from build123d import *

# Parameters (mm, degrees)
ESQUISSE1_R                             = 3
BOSS_EXTRU_1_DEPTH                      = 27
DIAM_TRE_DU_PER_AGE_3_0_3_1_D           = 3
DIAM_TRE_DU_PER_AGE_3_0_3_1_DEPTH       = 24.5
DIAM_TRE_DU_PER_AGE_3_0_3_1_CSINK_D     = 3.05
DIAM_TRE_DU_PER_AGE_3_0_3_1_CSINK_ANGLE = 90
DIAM_TRE_DU_PER_AGE_3_0_3_1_TIP         = 0.901290929
DIAM_TRE_DU_PER_AGE_2_5_2_5_1_D         = 2.5
DIAM_TRE_DU_PER_AGE_2_5_2_5_1_DEPTH     = 2.5
DIAM_TRE_DU_PER_AGE_2_5_2_5_1_TIP       = 0.751075774
ENL_V_START                             = -15
ESQUISSE8_W                             = 10.37088702
ESQUISSE8_H                             = 7.120487756
ESQUISSE8_R                             = 2.25
ENL_V_MAT_EXTRU_1_DEPTH                 = 6
CHANFREIN1_SIZE                         = 1
CHANFREIN2_SIZE                         = 0.75


with BuildPart() as part:
    # Esquisse1 → Boss.-Extru.1 (new body)
    with BuildSketch(Plane.XY):
        Circle(ESQUISSE1_R)
    extrude(amount=BOSS_EXTRU_1_DEPTH)

    # Diamètre du perçage Ø3.0 (3)1
    with Locations(Plane.XY.offset(27)):
        with Locations((0, 0)):
            CounterSinkHole(DIAM_TRE_DU_PER_AGE_3_0_3_1_D / 2, DIAM_TRE_DU_PER_AGE_3_0_3_1_CSINK_D / 2, depth=DIAM_TRE_DU_PER_AGE_3_0_3_1_DEPTH, counter_sink_angle=DIAM_TRE_DU_PER_AGE_3_0_3_1_CSINK_ANGLE)
            with Locations((0, 0, -(DIAM_TRE_DU_PER_AGE_3_0_3_1_DEPTH + DIAM_TRE_DU_PER_AGE_3_0_3_1_TIP / 2))):  # 118° drill point
                Cone(0, DIAM_TRE_DU_PER_AGE_3_0_3_1_D / 2, DIAM_TRE_DU_PER_AGE_3_0_3_1_TIP, mode=Mode.SUBTRACT)

    # Diamètre du perçage Ø2.5 (2.5)1
    with Locations(Plane(origin=(0, 0, 0), x_dir=(-1, 0, 0), z_dir=(0, 0, -1))):
        with Locations((0, 0)):
            Hole(DIAM_TRE_DU_PER_AGE_2_5_2_5_1_D / 2, depth=DIAM_TRE_DU_PER_AGE_2_5_2_5_1_DEPTH)
            with Locations((0, 0, -(DIAM_TRE_DU_PER_AGE_2_5_2_5_1_DEPTH + DIAM_TRE_DU_PER_AGE_2_5_2_5_1_TIP / 2))):  # 118° drill point
                Cone(0, DIAM_TRE_DU_PER_AGE_2_5_2_5_1_D / 2, DIAM_TRE_DU_PER_AGE_2_5_2_5_1_TIP, mode=Mode.SUBTRACT)

    # Esquisse8 → Enlèv. mat.-Extru.1 (cut)
    with BuildSketch(Plane.XY.offset(27).offset(ENL_V_START)):
        with Locations((-0.50743182, -0.050962128)):
            Rectangle(ESQUISSE8_W, ESQUISSE8_H)
        Circle(ESQUISSE8_R, mode=Mode.SUBTRACT)
    extrude(amount=-ENL_V_MAT_EXTRU_1_DEPTH, mode=Mode.SUBTRACT)

    # Chanfrein1
    chanfrein1_edges = [part.edges().sort_by_distance(p)[0] for p in [
        (-3, 0, 0),
    ]]
    chamfer(chanfrein1_edges, length=CHANFREIN1_SIZE)

    # Chanfrein2
    chanfrein2_edges = [part.edges().sort_by_distance(p)[0] for p in [
        (-2.25, 0, 6),
    ]]
    chamfer(chanfrein2_edges, length=CHANFREIN2_SIZE - 0.0001)  # a hair under: the kernel refuses the full size


solid = part.part
Can you work these out from the model? Positions are in its coordinate system, mm. A direction names the side the tool comes from. Round coordinates to 2 decimals unless told otherwise and drop trailing zeros. Loops run counter-clockwise (first coordinate to the right, second up) from the corner with the lowest first, then second, coordinate; pieces in that order, holes last. Notation, with made-up numbers: (-4.75, 72.5) - (26.25, 72.5) arc R19 cw to (26.25, 92.5) - close; hole circle Ø2 at (60.25, 83.25). An arc over 180 degrees is marked (long way). Write item = value, one per line. Start each with the question number.
(1) If I drill on probe 1 along Y at (x, z) = (0, 20); probe 2 along Y at (x, z) = (0, 1.4), over which ranges is the centre line in solid material (lowest first)? Write a range as [from, to].
(2) For P1, Ø1.5, axis at x = 2, z = 12.5, coming from the -Y side; P2, Ø3, axis at y = 2, z = 14.5, coming from the +X side, each with a flat end and sliding along its axis, tell me the tip position at first contact or that it passes through.
(3) If we mould it in two halves opening along Z, with no side actions, what happens to faces 1 (the face through (-0.29, 2.23, 9.41)), 2 (the face through (1, 1, 0)), 3 (the face through (1.3, -1.3, 27)), 4 (the face through (-3, 0, 19))? For each: released by +Z, released by -Z, zero draft, split by the parting line, or undercut.
(4) If we section it at D-D (z = 9.25): Please give me the cut outline in (x, y).
(5) For faces 5 (the face through (1.5, 0.07, 14.57)), 6 (the face through (-3, 0, 3)), which set-ups out of +Z, -Z, +X, -X, +Y, -Y let a thin tool reach every point of the face, with its end or its side?
(6) If we section it at C-C (z = 19.5): Please give me the cut outline in (x, y).
Ans:
q1.probe_1 = [-3, -1.5], [1.5, 3]
q1.probe_2 = [-3, -1.25], [1.25, 3]
q2.P1 = -2.73
q2.P2 = 2.96
q3.face_1 = undercut
q3.face_2 = released by -Z
q3.face_3 = released by +Z
q3.face_4 = zero draft
q4.outline = circle Ø4.5 at (0, 0); hole circle Ø3 at (0, 0)
q5.face_5 = +Z
q5.face_6 = +Z, -Z
q6.outline = circle Ø6 at (0, 0); hole circle Ø3 at (0, 0)
